```python
from build123d import *

# Parameters (mm, degrees)
SKETCH_1_W          = 100
SKETCH_1_H          = 40
EXTRUDE_1_DEPTH     = 3
SKETCH_6_R          = 1.4
CUT_EXTRUDE_4_DEPTH = 3
SKETCH_7_W          = 60
SKETCH_7_H          = 20
CUT_EXTRUDE_5_DEPTH = 3
SKETCH_8_R          = 3
SKETCH_8_R_2        = 6.5
SKETCH_8_R_3        = 1.1
CUT_EXTRUDE_6_DEPTH = 3
FILLET_1_R          = 10


with BuildPart() as part:
    # 草图1 → 凸台-拉伸1 (new body)
    with BuildSketch(Plane.XY):
        with Locations((50, 20)):
            Rectangle(SKETCH_1_W, SKETCH_1_H)
    extrude(amount=EXTRUDE_1_DEPTH)

    # 草图6 → 切除-拉伸4 (cut)
    with BuildSketch(Plane(origin=(0, 0, 0), x_dir=(-1, 0, 0), z_dir=(0, 0, -1))):
        with Locations((-20, 5)):
            Circle(SKETCH_6_R)
        with Locations((-20, 17)):
            Circle(SKETCH_6_R)
        with Locations((-33, 17)):
            Circle(SKETCH_6_R)
        with Locations((-33, 5)):
            Circle(SKETCH_6_R)
    extrude(amount=-CUT_EXTRUDE_4_DEPTH, mode=Mode.SUBTRACT)

    # 草图7 → 切除-拉伸5 (cut)
    with BuildSketch(Plane.XY.offset(3)):
        with Locations((70, 10)):
            Rectangle(SKETCH_7_W, SKETCH_7_H)
    extrude(amount=-CUT_EXTRUDE_5_DEPTH, mode=Mode.SUBTRACT)

    # 草图8 → 切除-拉伸6 (cut)
    with BuildSketch(Plane.XY.offset(3)):
        with Locations((19.54, 31)):
            Circle(SKETCH_8_R)
        with Locations((13.54, 31)):
            Circle(SKETCH_8_R_2)
        with Locations((5, 31)):
            Circle(SKETCH_8_R_3)
        with Locations((32.68, 31)):
            Circle(SKETCH_8_R_3)
    extrude(amount=-CUT_EXTRUDE_6_DEPTH, mode=Mode.SUBTRACT)

    # 圆角1
    fillet_1_edges = [part.edges().sort_by_distance(p)[0] for p in [
        (0, 40, 1.5),
        (100, 40, 1.5),
        (0, 0, 1.5),
    ]]
    fillet(fillet_1_edges, radius=FILLET_1_R)


solid = part.part
```
Design review of the part built by this model. Coordinates are the model's own, in mm. A direction names the side the tool comes from. Coordinates: 2 decimals unless noted, no trailing zeros. Order: outer loops, then holes, each group sorted by start corner. A loop starts at its lowest first (then second) coordinate and runs counter-clockwise, first axis right, second up.
1) Mouldability with a two-part tool opening along Y and no side actions: class faces 3 (the flat face through (40, 10, 2)), 4 (the flat face through (70, 20, 2)), 5 (the cylindrical face through (34.4, 17.06, 1.48)), 6 (the cylindrical face through (21.03, 5.95, 1.48)) as +Y half, -Y half, draft (parallel to the pull), parting line (faces both ways), or undercut.
2) Take a section at D-D, the plane z = 1.4. Give the boundary of the cut face in (x, y), and give its area (3 significant figures).
3) Take a section at B-B, the plane y = 29. Give the boundary of the cut face in (x, z).
4) Take a section at A-A, the plane x = 13.54. Give the boundary of the cut face in (y, z).
5) Take a section at C-C, the plane x = 32.68. Give the boundary of the cut face in (y, z), and give its area (3 significant figures).
6) Wall thickness on line 1 along X through (y, z) = (18, 1.4); line 2 along Y through (x, z) = (13.54, 2); line 3 along Y through (x, z) = (73, 1.1): over which ranges is each line inside the solid? List them lowest first.
7) For faces 1 (the flat face through (38, 25, 3)), 2 (the cylindrical face through (22.54, 30.93, 1.52)), list the 3-axis set-ups (+Z, -Z, +X, -X, +Y, -Y) from which the entire face can be reached by the end or side of a thin tool; tool diameter is ignored.
8) Clearance check with a flat-ended pin moving along its axis: pin 1 (1.5 mm diameter, centred on x = 78.5, z = 1, fed in from -Y). State where the tip first meets the part, or that it passes through.
Returned:
1. face 3: draft
1. face 4: -Y half
1. face 5: undercut
1. face 6: undercut
2. outline: (0, 10) arc R10 ccw to (10, 0) - (40, 0) - (40, 20) - (100, 20) - (100, 30) arc R10 ccw to (90, 40) - (10, 40) arc R10 ccw to (0, 30) - close; hole circle Ø2.2 at (5, 31); hole circle Ø2.8 at (20, 5); hole circle Ø2.8 at (20, 17); hole (19.31, 28.01) arc R3 ccw (long way) to (19.31, 33.99) arc R6.5 ccw (long way) to start; hole circle Ø2.2 at (32.68, 31); hole circle Ø2.8 at (33, 5); hole circle Ø2.8 at (33, 17)
2. area: 2,560 mm2
3. outline: (0, 0) - (7.36, 0) - (7.36, 3) - (0, 3) - close; (21.78, 0) - (100, 0) - (100, 3) - (21.78, 3) - close
4. outline: (0, 0) - (24.5, 0) - (24.5, 3) - (0, 3) - close; (37.5, 0) - (40, 0) - (40, 3) - (37.5, 3) - close
5. outline: (0, 0) - (3.64, 0) - (3.64, 3) - (0, 3) - close; (6.36, 0) - (15.64, 0) - (15.64, 3) - (6.36, 3) - close; (18.36, 0) - (29.9, 0) - (29.9, 3) - (18.36, 3) - close; (32.1, 0) - (40, 0) - (40, 3) - (32.1, 3) - close
5. area: 97.0 mm2
6. line 1: x = 0 to 19.02, 20.98 to 32.02, 33.98 to 40
6. line 2: y = 0 to 24.5, 37.5 to 40
6. line 3: y = 20 to 40
7. face 1: +Z, +X, -X, +Y, -Y
7. face 2: +Z, -Z
8. pin 1: stops at y = 20
